Build history of the part. All positions in model axes, mm. A direction names the side the tool comes from. Round coordinates to 2 decimals unless told otherwise and drop trailing zeros. Order: outer loops, then holes, each group sorted by start corner. A loop starts at its lowest first (then second) coordinate and runs counter-clockwise, first axis right, second up. Notation, with made-up numbers: M 69,-27 L 87,-27 A18 cw 87,0 Z; hole C 54,-17 d2. An arc over 180 degrees is marked long. One line per item, written item: value. Start each with the question number.
Item 1: Tool access for faces 4 (the flat face through (17, 0, -17)), 5 (the cylindrical face through (23.846, -39.72, 7.509)), 6 (the cylindrical face through (-8.67, -9.86, -39.05)): list every direction of +Z, -Z, +X, -X, +Y, -Y with a clear straight run to the whole face (end or side of a thin tool).
Item 2: Probe L1, parallel to Z at x = 0, y = -42; L2, parallel to X at y = -19.5, z = -1.5; L3, parallel to X at y = -30, z = 17.5. List the from-to ranges inside material, lowest first.
Item 3: Band-saw the part on C-C, the plane y = 89. Write the cut outline in (x, z).
Item 4: Pin check, flat tips, straight feed: pin 1 (12 mm diameter, centred on x = -8, z = -9, fed in from +Y); pin 2 (12 mm diameter, centred on x = -9, y = -3, fed in from -Z); pin 3 (4 mm diameter, centred on x = -0.5, z = -9.5, fed in from -Y). Stop position of each tip, or through.
Item 5: Band-saw the part on B-B, the plane y = 64.5. Write the cut outline in (x, z).
Item 6: Band-saw the part on D-D, the plane x = 17. Write the cut outline in (y, z), then the cut area to 3 significant figures.
Item 7: Band-saw the part on A-A, the plane x = 32. Write the cut outline in (y, z).
Item 8: Two-plate mould, pull along X, no slides. Class faces 1 (the cylindrical face through (14.985, 49.86, 0.66)), 2 (the flat face through (-3, 60, -10)), 3 (the cylindrical face through (-4.336, -40.28, -19.524)): +X half, -X half, draft (parallel to the pull), parting line (faces both ways), or undercut.
```python
from build123d import *

# Parameters (mm, degrees)
F0_R      = 40
F1_DEPTH  = 20
F2_R      = 25
F3_DEPTH  = 40
F4_R      = 20
F5_DEPTH  = 40
F6_R      = 22.1974572785
F7_DEPTH  = 20
F8_R      = 20
F9_DEPTH  = 20
F10_R     = 15
F11_DEPTH = 20
F12_R     = 10
F13_DEPTH = 20
F14_R     = 5
F15_DEPTH = 20
F16_R     = 2.5
F17_DEPTH = 20


with BuildPart() as f1:
    # F0 (on Front) → F1 (new body)
    with BuildSketch(Plane.XZ):
        Circle(F0_R)
    extrude(amount=F1_DEPTH)

    # F2 (on face) → F3 (join)
    with BuildSketch(Plane.XZ.offset(20)):
        Circle(F2_R)
    extrude(amount=F3_DEPTH)

    # F4 (on face) → F5 (cut)
    with BuildSketch(Plane.XZ.offset(60)):
        Circle(F4_R)
    extrude(amount=-F5_DEPTH, mode=Mode.SUBTRACT)

    # F6 (on face) → F7 (join)
    with BuildSketch(Plane(origin=(0, 0, 0), x_dir=(-1, 0, 0), z_dir=(0, 1, 0))):
        Circle(F6_R)
    extrude(amount=F7_DEPTH)

    # F8 (on face) → F9 (join)
    with BuildSketch(Plane(origin=(0, 20, 0), x_dir=(-1, 0, 0), z_dir=(0, 1, 0))):
        Circle(F8_R)
    extrude(amount=F9_DEPTH)

    # F10 (on face) → F11 (join)
    with BuildSketch(Plane(origin=(0, 40, 0), x_dir=(-1, 0, 0), z_dir=(0, 1, 0))):
        Circle(F10_R)
    extrude(amount=F11_DEPTH)

    # F12 (on face) → F13 (join)
    with BuildSketch(Plane(origin=(0, 60, 0), x_dir=(-1, 0, 0), z_dir=(0, 1, 0))):
        Circle(F12_R)
    extrude(amount=F13_DEPTH)

    # F14 (on face) → F15 (join)
    with BuildSketch(Plane(origin=(0, 80, 0), x_dir=(-1, 0, 0), z_dir=(0, 1, 0))):
        Circle(F14_R)
    extrude(amount=F15_DEPTH)

    # F16 (on face) → F17 (join)
    with BuildSketch(Plane(origin=(0, 100, 0), x_dir=(-1, 0, 0), z_dir=(0, 1, 0))):
        Circle(F16_R)
    extrude(amount=F17_DEPTH)


solid = f1.part
```
Output:
1. face 4: +Y
1. face 5: -Y
1. face 6: +Y, -Y
2. L1: z = -25 to -20, 20 to 25
2. L2: x = -39.97 to 39.97
2. L3: x = -17.85 to -9.68, 9.68 to 17.85
3. outline: C 0,0 d10
4. pin 1: stops at y = 80
4. pin 2: stops at z = -39.89
4. pin 3: stops at y = -20
5. outline: C 0,0 d20
6. outline: M -60,-18.33 L -20,-18.33 L -20,-36.21 L 0,-36.21 L 0,-14.27 L 20,-14.27 L 20,-10.54 L 40,-10.54 L 40,10.54 L 20,10.54 L 20,14.27 L 0,14.27 L 0,36.21 L -20,36.21 L -20,18.33 L -60,18.33 L -60,10.54 L -20,10.54 L -20,-10.54 L -60,-10.54 Z
6. area: 3,060 mm²
7. outline: M -20,-24 L 0,-24 L 0,24 L -20,24 Z
8. face 1: parting line
8. face 2: draft
8. face 3: undercut
